Design review of the part built by this model. Coordinates are the model's own, in mm. Face numbers are marked on the shaded views. Round coordinates to 2 decimals unless told otherwise and drop trailing zeros. Order: outer loops, then holes, each group sorted by start corner. A loop starts at its lowest first (then second) coordinate and runs counter-clockwise, first axis right, second up. Notation, with made-up numbers: (38.5, 10.25) - (87.5, 10.25) arc R28 cw to (87.5, 31.25) - close; hole circle Ø5 at (20, 32). An arc over 180 degrees is marked (long way). Answer as a JSON object with one key per item and string values. Group by question number.
from build123d import *

# Parameters (mm, degrees)
SKETCH1_W              = 51
SKETCH1_H              = 32
BOSS_EXTRUDE1_DEPTH    = 4.5
FILLET1_R              = 0.5
LPATTERN1_COUNT        = 8
LPATTERN1_PITCH        = 5.8
FILLET1_OF_LPATTERN1_R = 0.5
M3X0_5_TAPPED_HOLE1_D  = 2.5


# Read off the part's stored shape, not the designer's step: Mirror1
with BuildPart() as part:
    # Sketch1 → Boss-Extrude1 (new body)
    with BuildSketch(Plane(origin=(0, 0, 0), x_dir=(1, 0, 0), z_dir=(0, 1, 0))):
        Rectangle(SKETCH1_W, SKETCH1_H)
    extrude(amount=-BOSS_EXTRUDE1_DEPTH)

    # Sketch2 → Loft1 section 0
    with BuildSketch(Plane(origin=(0, -4.5, 0), x_dir=(-1, 0, 0), z_dir=(0, -1, 0))):
        with BuildLine():
            Line((25.5, -16), (23.2, -16))
            Line((23.2, -16), (23.2, 16))
            Line((23.2, 16), (25.5, 16))
            Line((25.5, 16), (25.5, -16))
        make_face()
    # Sketch3 → Loft1 section 1
    with BuildSketch(Plane(origin=(0, -23, 0), x_dir=(1, 0, 0), z_dir=(0, 1, 0))):
        with BuildLine():
            Line((-23.6, -16), (-25.1, -16))
            Line((-25.1, -16), (-25.1, 16))
            Line((-25.1, 16), (-23.6, 16))
            Line((-23.6, 16), (-23.6, -16))
        make_face()
    loft1 = loft()

    # Fillet1
    fillet1_edges = [part.edges().sort_by_distance(p)[0] for p in [
        (-25.1, -23, 0),
        (-23.6, -23, 0),
    ]]
    fillet(fillet1_edges, radius=FILLET1_R)

    # LPattern1: Loft1 ×8
    with Locations(*[(i * LPATTERN1_PITCH, 0, 0) for i in range(1, LPATTERN1_COUNT)]):
        add(loft1)

    # Fillet1 of LPattern1
    fillet1_of_lpattern1_edges = [part.edges().sort_by_distance(p)[0] for p in [
        (-19.3, -23, 0),
        (-17.8, -23, 0),
        (-13.5, -23, 0),
        (-12, -23, 0),
        (-7.7, -23, 0),
        (-6.2, -23, 0),
        (-1.9, -23, 0),
        (-0.4, -23, 0),
        (3.9, -23, 0),
        (5.4, -23, 0),
        (9.7, -23, 0),
        (11.2, -23, 0),
        (15.5, -23, 0),
        (17, -23, 0),
    ]]
    fillet(fillet1_of_lpattern1_edges, radius=FILLET1_OF_LPATTERN1_R)

    # Sketch5 → Loft2 section 0
    with BuildSketch(Plane(origin=(0, -23, 0), x_dir=(1, 0, 0), z_dir=(0, 1, 0))):
        with BuildLine():
            Line((25.5, -16), (21.5, -16))
            Line((21.5, -16), (21.5, 16))
            Line((21.5, 16), (25.5, 16))
            Line((25.5, 16), (25.5, -16))
        make_face()
    # Sketch4 → Loft2 section 1
    with BuildSketch(Plane(origin=(0, -4.5, 0), x_dir=(-1, 0, 0), z_dir=(0, -1, 0))):
        with BuildLine():
            Line((-25.5, -16), (-20.5, -16))
            Line((-20.5, -16), (-20.5, 16))
            Line((-20.5, 16), (-25.5, 16))
            Line((-25.5, 16), (-25.5, -16))
        make_face()
    loft()

    # M3x0.5 Tapped Hole1 (through all)
    with Locations(Plane(origin=(0, 0, 0), x_dir=(1, 0, 0), z_dir=(0, 1, 0))):
        with Locations((13.5, 0)):
            Hole(M3X0_5_TAPPED_HOLE1_D / 2)

    # Mirror1 outline → Mirror1 (revolve, cut)
    with BuildSketch(Plane(origin=(-13.5, 0, 0), x_dir=(1, 0, 0), z_dir=(0, 0, 1))):
        Polygon((0, 0), (0, -5.251075774), (1.250000005, -4.499999997), (1.25, 0), align=None)
    revolve(axis=Axis((-13.5, 0, 0), (0, 1, 0)), mode=Mode.SUBTRACT)


solid = part.part
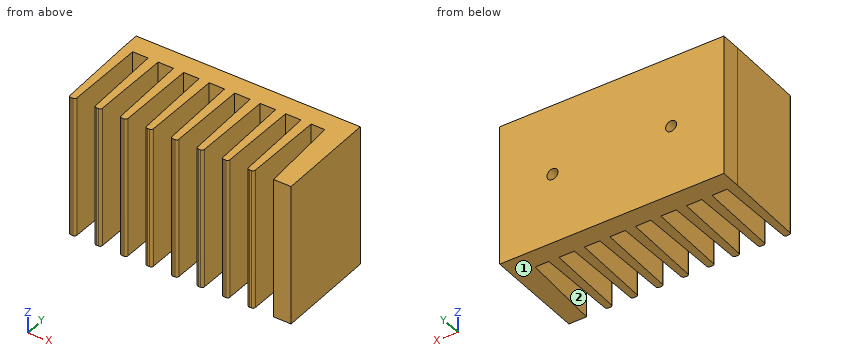
1. Clearance check with flat-ended pins moving along their axes: P1, Ø1.8, axis at x = 13.5, z = -5, coming from the -Y side; P2, Ø1, axis at x = 11.5, z = -7.5, coming from the -Y side; P3, Ø5, axis at y = -16.5, z = 5, coming from the -X side; P4, Ø6, axis at x = 19.5, z = 6, coming from the +Y side. State where each tip first meets the part, or that it passes through.
2. Mouldability with a two-part tool opening along X and no side actions: class the marked faces 1 and 2 as pulls with the +X half, pulls with the -X half, needs draft (parallel to the pull), parting line crosses it, or undercut.
3. Take a section at B-B, the plane y = -14.25. Count the separate pieces of the cut face and the enclosed holes in it, then the cut area to 3 significant figures.
4. Take a section at A-A, the plane x = 13.5. Give the boundary of the cut face in (y, z).
5. To check wall thickness, follow line 1 (Z direction, x = 13.5, y = -3.3); line 2 (Y direction, x = 18, z = -3); line 3 (Y direction, x = -19, z = -6.5). State the ranges of each line that lie inside material, in increasing order. Write a range as from..to.
Response values:
{
 "1": {"P1": "y = -4.5", "P2": "y = -22.91", "P3": "x = -25.29", "P4": "y = 0"},
 "2": {"face 1": "needs draft", "face 2": "undercut"},
 "3": {"separate pieces": "9", "enclosed holes": "0", "area": "624 mm2"},
 "4": {"outline": "(-4.5, -16) - (0, -16) - (0, -1.25) - (-4.5, -1.25) - close; (-4.5, 1.25) - (0, 1.25) - (0, 16) - (-4.5, 16) - close"},
 "5": {"line 1": "-16..-1.25, 1.25..16", "line 2": "-4.5..0", "line 3": "-22.96..0"}
}
